Design review of the part built by this model. Coordinates are the model's own, in mm. A direction names the side the tool comes from. Coordinates: 2 decimals unless noted, no trailing zeros. Write each loop counter-clockwise with the first axis right and the second up, starting at its lowest first coordinate (ties: lowest second). Pieces come first, ordered by that corner, then holes. Notation, with made-up numbers: (70.25, 72.5) -> (126.25, 72.5) arc R24 cw to (126.25, 83.5) -> close; hole circle Ø9 at (48.5, -29.5). An arc over 180 degrees is marked (long way). Write item = value, one per line. Start each with the question number.
Autodesk Inventor part; units mm, degrees
ref_plane "Plan de construction2" through (-24.996, -18.6052, -16) normal (0, 0, -1) x (0, 1, 0)
ref_plane "Plan de construction3" through (-23.77, -32.9273, -21) normal (0, 0, -1) x (0, 1, 0)
ref_plane "YZ Plane" through (0, 0, 0) normal (1, 0, 0) x (0, 1, 0)
ref_plane "Plan de construction1" through (0, 0, 0) normal (0, 0, 1) x (1, 0, 0)
sketch "Esquisse1" plane through (0, 0, 0) normal (0, 0, 1) x (1, 0, 0)
  circle A0 centre (18, -9.1573) radius 3.05
  arc A1 (16.3537, 35.0227) -> (19.3537, 33.6971) centre (18.8691, 36.6577) ccw
  arc A2 (16.3537, 35.0227) -> (9.6181, 34.9787) centre (13, 32.8427) ccw
  arc A3 (6.0453, 33.7654) -> (9.6181, 34.9787) centre (7.0816, 36.5807) ccw
  arc A4 (6.0453, 33.7654) -> (-6.0453, 33.7654) centre (0, 17.3427) ccw
  arc A5 (-9.6181, 34.9787) -> (-6.0453, 33.7654) centre (-7.0816, 36.5807) ccw
  arc A6 (-9.6181, 34.9787) -> (-16.3537, 35.0227) centre (-13, 32.8427) ccw
  arc A7 (-19.3537, 33.6971) -> (-16.3537, 35.0227) centre (-18.8691, 36.6577) ccw
  arc A8 (-19.3537, 33.6971) -> (-23.0131, 27.1188) centre (-20, 29.7497) ccw
  line L0 (-23.0131, 27.1188) -> (-21.6977, 25.6123)
  arc A9 (-21.984, 21.3792) -> (-21.6977, 25.6123) centre (-23.9573, 23.6389) ccw
  line L1 (-21.984, 21.3792) -> (-23.6265, 19.9451)
  arc A10 (-23.6265, 19.9451) -> (-23.5067, 13.8184) centre (-20.9956, 16.932) ccw
  arc A11 (-20.4202, 0.2907) -> (-23.5067, 13.8184) centre (-30.5395, 5.0978) ccw
  arc A12 (-20.4202, 0.2907) -> (-21.1202, -16.9153) centre (0, -9.1573) ccw
  line L2 (-21.1202, -16.9153) -> (-25.0562, -21.5766)
  arc A13 (-25.0562, -21.5766) -> (-25.898, -25.0549) centre (-22, -24.1573) ccw
  line L3 (-25.898, -25.0549) -> (-23.898, -33.7403)
  arc A14 (-23.898, -33.7403) -> (-16.9438, -35.4234) centre (-20, -32.8427) ccw
  line L4 (-16.9438, -35.4234) -> (-12.7634, -30.4726)
  arc A15 (-9.2394, -29.6727) -> (-12.7634, -30.4726) centre (-10.4713, -32.4081) ccw
  arc A16 (-9.2394, -29.6727) -> (9.2394, -29.6727) centre (0, -9.1573) ccw
  arc A17 (12.7634, -30.4726) -> (9.2394, -29.6727) centre (10.4713, -32.4081) ccw
  line L5 (12.7634, -30.4726) -> (16.9438, -35.4234)
  arc A18 (16.9438, -35.4234) -> (23.898, -33.7403) centre (20, -32.8427) ccw
  line L6 (23.898, -33.7403) -> (25.898, -25.0549)
  arc A19 (25.898, -25.0549) -> (25.0562, -21.5766) centre (22, -24.1573) ccw
  line L7 (25.0562, -21.5766) -> (21.1202, -16.9153)
  arc A20 (21.1202, -16.9153) -> (20.477, 0.167) centre (0, -9.1573) ccw
  arc A21 (23.6268, 14.7402) -> (20.477, 0.167) centre (31.8353, 5.339) ccw
  arc A22 (23.6268, 14.7402) -> (23.507, 20.8669) centre (20.996, 17.7533) ccw
  line L8 (23.507, 20.8669) -> (22.4423, 21.7255)
  arc A23 (22.0658, 26.0339) -> (22.4423, 21.7255) centre (24.3256, 24.0608) ccw
  line L9 (22.0658, 26.0339) -> (23.0131, 27.1188)
  arc A24 (23.0131, 27.1188) -> (19.3537, 33.6971) centre (20, 29.7497) ccw
  circle A25 centre (13, 32.8427) radius 2
  circle A26 centre (-13, 32.8427) radius 2
  circle A27 centre (-22, -24.1573) radius 2
  circle A28 centre (22, -24.1573) radius 2
  circle A29 centre (-18, -9.1573) radius 3.05
  line L10 (0, -31.6573) -> (13.7637, -31.6573)
  line L11 (13.7637, -31.6573) -> (18.1423, -36.8427)
  line L12 (18.1423, -36.8427) -> (23.1836, -36.8427)
  line L13 (23.1836, -36.8427) -> (26.3469, -23.1052)
  line L14 (26.3469, -23.1052) -> (22.5, -18.5494)
  line L15 (22.5, -18.5494) -> (22.5, 13.6223)
  line L16 (22.5, 13.6223) -> (24.996, 16.0767)
  line L17 (24.996, 16.0767) -> (24.996, 31.9152)
  line L18 (24.996, 31.9152) -> (13.8443, 36.8427)
  line L19 (13.8443, 36.8427) -> (0, 36.8427)
  line L20 (0, 0) -> (0, -45.3526)
  line L21 (0, -31.6573) -> (-13.7637, -31.6573)
  line L22 (-13.7637, -31.6573) -> (-18.1423, -36.8427)
  line L23 (-18.1423, -36.8427) -> (-23.1836, -36.8427)
  line L24 (-23.1836, -36.8427) -> (-26.3469, -23.1052)
  line L25 (-26.3469, -23.1052) -> (-22.5, -18.5494)
  line L26 (-22.5, -18.5494) -> (-22.5, 13.6223)
  line L27 (-22.5, 13.6223) -> (-24.996, 16.0767)
  line L28 (-24.996, 16.0767) -> (-24.996, 31.9152)
  line L29 (-24.996, 31.9152) -> (-13.8443, 36.8427)
  line L30 (-13.8443, 36.8427) -> (0, 36.8427)
  point P0 (23.898, -33.7403)
ref_plane "Plan de construction2" through (-24.996, -18.6052, -16) normal (0, 0, -1) x (0, 1, 0)
extrude "Extrusion1" add sketch "Esquisse1" against normal up to surface (16 mm away) contours A0 | A2 L18 A24 A1 | A1 A24 L9 A23 L8 A22 A21 A20 L7 A19 L6 A18 L5 A17 A16 A15 L4 A14 L3 A13 L2 A12 A11 L26 L27 A10 L1 A9 L0 A8 A7 A6 A5 A4 A3 A2 | A2 L19 L18 | L18 L17 A22 L8 A23 L9 A24 | A2 A3 A4 A5 A6 L30 L19 | L17 L16 A22 | A6 L29 L30 | L16 A21 A22 | A6 A7 A8 L29 | L15 A20 A21 | A8 L0 A9 L1 A10 L28 L29 | L15 L7 A20 | A10 L27 L28 | L14 L13 A19 | L13 L12 A18 | A11 A12 L26 | L12 L11 A18 | A12 L2 L26 | L10 A16 A17 L5 | A13 L24 L25 | L21 L4 A15 A16 | A14 L23 L24 | L22 L23 A14 | A25 | A26 | A27 | A28 | A29
sketch "Esquisse2" plane through (0, -9.1573, -16) normal (0, 0, -1) x (-1, 0, 0)
  circle A0 centre (0, 0) radius 22.5035
  point P0 (0, 9.1573)
ref_plane "Plan de construction3" through (-23.77, -32.9273, -21) normal (0, 0, -1) x (0, 1, 0)
extrude "Extrusion2" add sketch "Esquisse2" along normal up to surface (5 mm away)
sketch "Esquisse3" plane through (0, -9.1573, -21) normal (0, 0, -1) x (-1, 0, 0)
  circle A0 centre (0, 0) radius 19.6378
  point P0 (0, 9.1573)
extrude "Extrusion3" add sketch "Esquisse3" along normal up to surface (41.2635 mm away)
properties part number "simple_lidar_shape"
(1) Take a section at B-B, the plane x = -9. State the section outline as (y, z) points, then the cut area to 3 significant figures.
(2) Take a section at A-A, the plane y = -11. State the section outline as (x, z) points, then the cut area to 3 significant figures.
(3) For pin 1 Ø13 at (x, z) = (2.5, -5) entering from -Y; pin 2 Ø1 at (x, y) = (19.5, 11.5) entering from -Z; pin 3 Ø2 at (y, z) = (-9, -51.5) entering from +X, all flat-tipped, find the tip position at first contact; note any pin that passes through.
(4) Mouldability with a two-part tool opening along Y and no side actions: class faces 5 (the face through (-21, -36.843, -8)), 6 (the face through (-24.996, 24, -8)), 7 (the face through (23.7, 14.8, -7.9)) as pulls with the +Y half, pulls with the -Y half, needs draft (parallel to the pull), parting line crosses it, or undercut.
(5) For line 1 (Z direction, x = -11.5, y = 32.5); line 2 (X direction, y = 5, z = -8.5); line 3 (Y direction, x = -23, z = -3.5), list the stretches that pass through material, from the lowest coordinate up.
(6) Take a section at D-D, the plane x = 21.5. State the section outline as (y, z) points, then the cut area to 3 significant figures.
(7) Take a section at C-C, the plane z = -33. State the section outline as (x, y) points.
(8) For faces 1 (the face through (19, -27, -16)), 2 (the face through (22.5, -3, -8)), 3 (the face through (-2, 11, -21)), 4 (the face through (0, -31.657, -8)), list the 3-axis set-ups (+Z, -Z, +X, -X, +Y, -Y) from which the entire face can be reached by the end or side of a thin tool; tool diameter is ignored.
Report:
q1.outline = (-31.66, -16) -> (-29.78, -16) -> (-29.78, -21) -> (-26.61, -21) -> (-26.61, -62.26) -> (8.3, -62.26) -> (8.3, -21) -> (11.47, -21) -> (11.47, -16) -> (36.84, -16) -> (36.84, 0) -> (-31.66, 0) -> close
q1.area = 2,740 mm2
q2.outline = (-22.5, -16) -> (-22.43, -16) -> (-22.43, -21) -> (-19.55, -21) -> (-19.55, -62.26) -> (19.55, -62.26) -> (19.55, -21) -> (22.43, -21) -> (22.43, -16) -> (22.5, -16) -> (22.5, 0) -> (-22.5, 0) -> close
q2.area = 2,560 mm2
q3.pin_1 = -31.66
q3.pin_2 = -16
q3.pin_3 = 19.64
q4.face_5 = pulls with the -Y half
q4.face_6 = needs draft
q4.face_7 = undercut
q5.line_1 = -16 to 0
q5.line_2 = -22.5 to 22.5
q5.line_3 = -36.84 to -19.14, 14.11 to 32.8
q6.outline = (-36.84, -16) -> (-15.8, -16) -> (-15.8, -21) -> (-2.51, -21) -> (-2.51, -16) -> (33.46, -16) -> (33.46, 0) -> (-36.84, 0) -> close
q6.area = 1,190 mm2
q7.outline = circle Ø39.28 at (0, -9.16)
q8.face_1 = -Z, +X, -Y
q8.face_2 = +Z, -Z, +X
q8.face_3 = -Z
q8.face_4 = +Z, -Z, -Y
